The listing builds one solid part. Answer for the finished solid, in the listing's coordinates (mm). A direction names the side the tool comes from. Round coordinates to 2 decimals unless told otherwise and drop trailing zeros. Order: outer loops, then holes, each group sorted by start corner. A loop starts at its lowest first (then second) coordinate and runs counter-clockwise, first axis right, second up. Notation, with made-up numbers: M -33,-1 L -5,-1 A23 ccw -5,29 Z; hole C 7.5,33 d2. An arc over 180 degrees is marked long. Put each result on its own line as item: value. Start each with the question number.
1. The part is cut by section B-B (x = 14). Give the vertices of the cut face in (y, z), then the cut area to 3 significant figures.
2. Consider line 1 (Z direction, x = 4, y = -47); line 2 (X direction, y = -40, z = -6); line 3 (Y direction, x = -5, z = 3). Determine where each line is inside the solid, lowest interval first.
3. This flat-tipped pin is pushed along its axis until it touches: pin 1 Ø12 at (x, z) = (-7.5, 0.5) entering from -Y. Where does it stop, or does it pass through?
4. The part is cut by section C-C (z = 11). Give the vertices of the cut face in (x, y), then the cut area to 3 significant figures.
5. The mould has two halves that part along Z. Classify faces 3 (the face through (0, 0, 0)), 4 (the face through (0, -31, -23.219)), 5 (the face through (18.698, -44, 0)): +Z half, -Z half, draft (parallel to the pull), parting line (faces both ways), or undercut.
6. The part is cut by section A-A (y = -27). Give the vertices of the cut face in (x, z), then the cut area to 3 significant figures.
7. Which of the six approach directions +Z, -Z, +X, -X, +Y, -Y give full straight-line access (tool end or side, diameter ignored) to faces 1 (the face through (31.455, -31, 0)), 2 (the face through (-18.698, -44, 0))?
from build123d import *

# Parameters (mm, degrees)
F0_W     = 62.910616
F0_H     = 46.43853
F0_W_2   = 37.395
F0_H_2   = 27.496278
F1_DEPTH = 62.186921
F2_W     = 37.666064
F2_H     = 27.62061
F3_DEPTH = 25.4


with BuildPart() as f1:
    # F0 (on Front) → F1 (new body)
    with BuildSketch(Plane.XZ):
        Rectangle(F0_W, F0_H)
        Rectangle(F0_W_2, F0_H_2, mode=Mode.SUBTRACT)
    extrude(amount=F1_DEPTH)

    # F2 (on Front) → F3 (join)
    with BuildSketch(Plane.XZ):
        Rectangle(F2_W, F2_H)
    extrude(amount=F3_DEPTH)


solid = f1.part
Resolved:
1. outline: M -62.19,-23.22 L 0,-23.22 L 0,23.22 L -62.19,23.22 L -62.19,13.75 L -25.4,13.75 L -25.4,-13.75 L -62.19,-13.75 Z
1. area: 1,880 mm2
2. line 1: -23.22 to -13.75, 13.75 to 23.22
2. line 2: -31.46 to -18.7, 18.7 to 31.46
2. line 3: -25.4 to 0
3. pin 1: y = -25.4
4. outline: M -31.46,-62.19 L -18.7,-62.19 L -18.7,-25.4 L 18.7,-25.4 L 18.7,-62.19 L 31.46,-62.19 L 31.46,0 L -31.46,0 Z
4. area: 2,540 mm2
5. face 3: draft
5. face 4: -Z half
5. face 5: undercut
6. outline: M -31.46,-23.22 L 31.46,-23.22 L 31.46,23.22 L -31.46,23.22 Z; hole M -18.7,-13.75 L 18.7,-13.75 L 18.7,13.75 L -18.7,13.75 Z
6. area: 1,890 mm2
7. face 1: +Z, -Z, +X, +Y, -Y
7. face 2: -Y
